Answer from the drawing. Dimensions are ordinates in mm from the lowest x, y and z of the part. A direction names the side the tool comes from. Give positions to 0.01 mm unless a question says otherwise; leave off trailing zeros. Loops run counter-clockwise (first coordinate to the right, second up) from the corner with the lowest first, then second, coordinate; pieces in that order, holes last. Notation, with made-up numbers: (70.5, 0) - (121.5, 0) arc R28 cw to (121.5, 36) - close; hole circle Ø10 at (26, -25.5). An arc over 180 degrees is marked (long way). One line per item, written item: value.
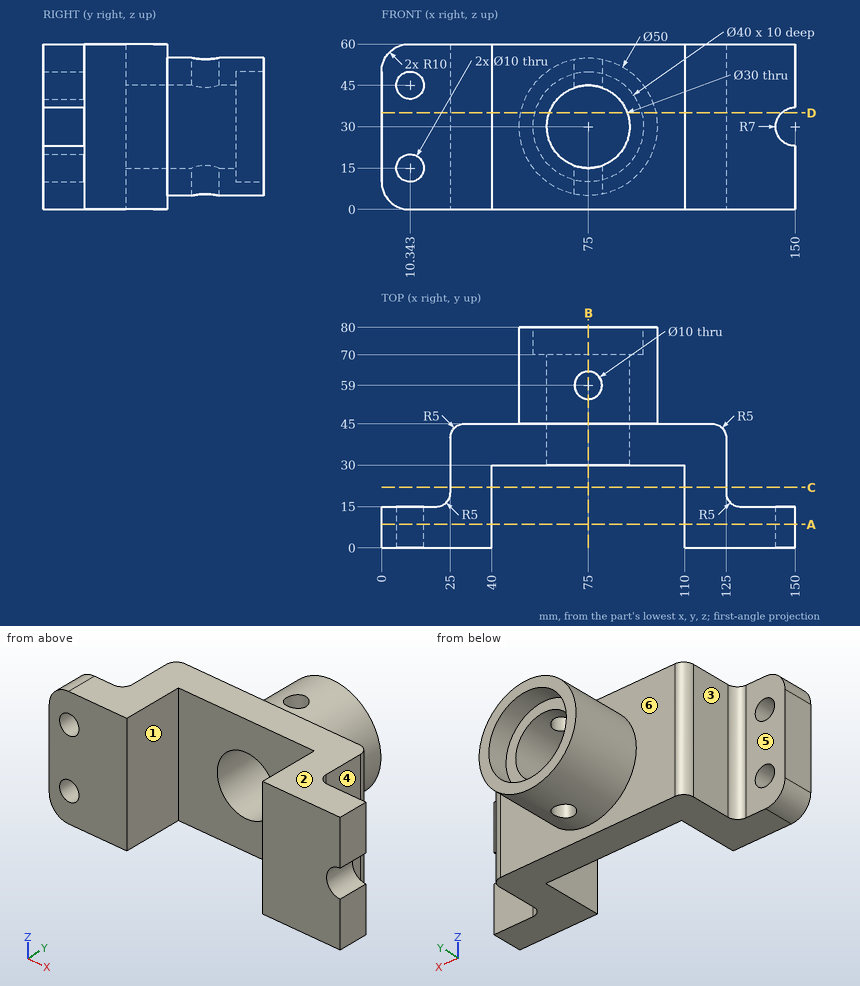
1. Section A-A (y = 8.5) is taken. Write down the section's boundary in (x, z), and give its area (3 significant figures).
Output:
outline: (0, 10) arc R10 ccw to (10, 0) - (40, 0) - (40, 60) - (10, 60) arc R10 ccw to (0, 50) - close; (110, 0) - (150, 0) - (150, 23) arc R7 cw to (150, 37) - (150, 60) - (110, 60) - close; hole circle Ø10 at (10.34, 15); hole circle Ø10 at (10.34, 45)
area: 4,520 mm²
2. Section B-B (x = 75) is taken. Write down the section's boundary in (y, z).
Output:
outline: (30, 0) - (45, 0) - (45, 5) - (54, 5) - (54, 15) - (30, 15) - close; (30, 45) - (54, 45) - (54, 55) - (45, 55) - (45, 60) - (30, 60) - close; (64, 5) - (80, 5) - (80, 10) - (70, 10) - (70, 15) - (64, 15) - close; (64, 45) - (70, 45) - (70, 50) - (80, 50) - (80, 55) - (64, 55) - close
3. Flat-ended cylindrical pins translate along their axes: pin 1 Ø12 at (y, z) = (40, 23) entering from -X; pin 2 Ø1 at (x, z) = (53, 17.5) entering from -Y; pin 3 Ø10 at (y, z) = (52.5, 15) entering from +X. Find the tip coordinate at first contact, or state that the pin passes through.
Output:
pin 1: stops at x = 25
pin 2: stops at y = 30
pin 3: stops at x = 97.91
4. Find the intervals of material crossed by line 1 along X through (y, z) = (27.5, 19.5); line 2 along Y through (x, z) = (75, 9.25); line 3 along Y through (x, z) = (86, 40.5), in increasing order.
Output:
line 1: x = 25 to 40, 110 to 125
line 2: y = 30 to 54, 64 to 80
line 3: y = 30 to 70
5. The mould has two halves that part along X. Classify the marked faces 1, 2 and 3: released by +X, released by -X, zero draft, split by the parting line, or undercut.
Output:
face 1: undercut
face 2: zero draft
face 3: released by -X
6. Section C-C (y = 22) is taken. Write down the section's boundary in (x, z).
Output:
outline: (25, 0) - (40, 0) - (40, 60) - (25, 60) - close; (110, 0) - (125, 0) - (125, 60) - (110, 60) - close
7. Section D-D (z = 35) is taken. Write down the section's boundary in (x, y) (1 decimal).
Output:
outline: (0, 0) - (40, 0) - (40, 30) - (60.9, 30) - (60.9, 70) - (55.6, 70) - (55.6, 80) - (50.5, 80) - (50.5, 45) - (30, 45) arc R5 ccw to (25, 40) - (25, 20) arc R5 cw to (20, 15) - (0, 15) - close; (89.1, 30) - (110, 30) - (110, 0) - (145.1, 0) - (145.1, 15) - (130, 15) arc R5 cw to (125, 20) - (125, 40) arc R5 ccw to (120, 45) - (99.5, 45) - (99.5, 80) - (94.4, 80) - (94.4, 70) - (89.1, 70) - close
8. For the marked faces 4, 5 and 6, determine the directions among +Z, -Z, +X, -X, +Y, -Y from which every point of the face is accessible in a straight line to the end or side of a thin tool.
Output:
face 4: +Z, -Z, +X, +Y
face 5: +Z, -Z, -X, +Y
face 6: +Y
